Could you check a few things on this model? Use its own coordinates, in mm. A direction names the side the tool comes from. Give positions to 0.01 mm unless a question says otherwise; leave off trailing zeros. Loops run counter-clockwise (first coordinate to the right, second up) from the corner with the lowest first, then second, coordinate; pieces in that order, holes last. Notation, with made-up numbers: (0.5, -32) -> (36.5, -32) arc R29 cw to (36.5, 7) -> close; hole circle Ø6 at (84, 6). An arc over 180 degrees is marked (long way). Write item = value, one per line. Start each with the question number.
1) If we mould it in two halves opening along X, with no side actions, what happens to faces 3 (the face through (26, 19.05, 9)), 4 (the face through (441, 50.8, 9))? For each: +X half, -X half, draft (parallel to the pull), parting line (faces both ways), or undercut.
2) I want a section at A-A (x = 589.5). List the corners of the cut face in (y, z) for me.
3) I'm going to push flat-ended pins straight in: pin 1 Ø6 at (x, z) = (131, 11.5) entering from +Y; pin 2 Ø5.5 at (x, z) = (29.5, 6.5) entering from +Y; pin 3 Ø1.5 at (x, z) = (92, 3.5) entering from -Y. Where does each tip first touch, or does it pass through?
4) On a 3-axis mill with a long thin cutter (end or side, diameter ignored), from which of +Z, -Z, +X, -X, +Y, -Y can I reach the whole of each face in a straight line? I mean faces 1 (the face through (864, 19.05, 9)), 2 (the face through (442, 58, 0)). Say none if no direction works.
5) I need wall thicknesses on probe 1 along Y at (x, z) = (398.5, 8); probe 2 along Y at (x, z) = (848, 2.75); probe 3 along X at (y, z) = (15.5, 16). Which ranges of each line are inside material? Lowest first, please. Write a range as from..to.
from build123d import *

# Parameters (mm, degrees)
F3_DEPTH = 19.05
F4_R     = 9.525
F5_R     = 254


# Not quite as in the source:
# - a variable given as a bare number and used for a length is read in inches; the dataset says mm whatever the document's units were


with BuildPart() as f3:
    # F2 (on Top) → F3 (new body)
    with BuildSketch(Plane.XY):
        Polygon((0, 19.05), (0, 0), (69.85, 0), (69.85, 50.8), (444.5, 50.8), (819.15, 50.8), (819.15, 0), (889, 0), (889, 19.05), (838.2, 19.05), (838.2, 69.85), (444.5, 69.85), (50.8, 69.85), (50.8, 19.05), align=None)
    extrude(amount=F3_DEPTH)

    # F4
    f4_edges = [f3.edges().sort_by_distance(p)[0] for p in [
        (69.85, 0, 9.525),
        (50.8, 19.05, 9.525),
        (819.15, 0, 9.525),
        (838.2, 19.05, 9.525),
        (0, 19.05, 9.525),
        (889, 19.05, 9.525),
    ]]
    fillet(f4_edges, radius=F4_R)

    # F5
    f5_edges = [f3.edges().sort_by_distance(p)[0] for p in [
        (69.85, 50.8, 9.525),
        (50.8, 69.85, 9.525),
        (819.15, 50.8, 9.525),
        (838.2, 69.85, 9.525),
    ]]
    fillet(f5_edges, radius=F5_R)


solid = f3.part
Answer list:
q1.face_3 = draft
q1.face_4 = undercut
q2.outline = (50.8, 0) -> (69.85, 0) -> (69.85, 19.05) -> (50.8, 19.05) -> close
q3.pin_1 = 61.96
q3.pin_2 = 19.05
q3.pin_3 = 18.13
q4.face_1 = +Z, -Z, +X, +Y
q4.face_2 = -Z, +X, -X, +Y, -Y
q5.probe_1 = 50.8..69.85
q5.probe_2 = 0..19.05
q5.probe_3 = 2.11..86.69, 802.31..886.89
